The figure shows three views and two pictorial views of one solid part (mm, origin at its lowest corner). Answer the questions. A direction names the side the tool comes from. Round coordinates to 2 decimals unless told otherwise and drop trailing zeros. Loops run counter-clockwise (first coordinate to the right, second up) from the corner with the lowest first, then second, coordinate; pieces in that order, holes last. Notation, with made-up numbers: (-27.5, 84.5) -> (11.5, 84.5) arc R26 cw to (11.5, 110.5) -> close; hole circle Ø1 at (29.25, -18). An arc over 180 degrees is marked (long way). Use a Markdown table: item, result. Add a question column.
Q1. For a pull along Y with two mould halves and no side action, classify the marked faces 1, 2 and 3 as released by +Y, released by -Y, zero draft, split by the parting line, or undercut.
Q2. Given pin 1 Ø1.5 at (x, z) = (2.5, 4) entering from -Y, flat-ended and moving along its own axis, determine where the tip first touches the part or whether it passes through.
Q3. Section A-A on y = 2.4 is taken. Give the vertices of the cut face in (x, z).
Q4. Which of the six approach directions +Z, -Z, +X, -X, +Y, -Y give full straight-line access (tool end or side, diameter ignored) to the marked faces 4 and 5?
Q5. Section C-C on z = 8.75 is taken. Give the vertices of the cut face in (x, y).
Q6. Section B-B on x = 3.15 is taken. Give the vertices of the cut face in (y, z).
Q7. Section D-D on x = 4.05 is taken. Give the vertices of the cut face in (y, z).
Q8. Consider line 1 (Z direction, x = 1.1, y = 4.2); line 2 (X direction, y = 1.8, z = 10.75); line 3 (Z direction, x = 2.2, y = 2.6). Determine where each line is inside the solid, lowest interval first.
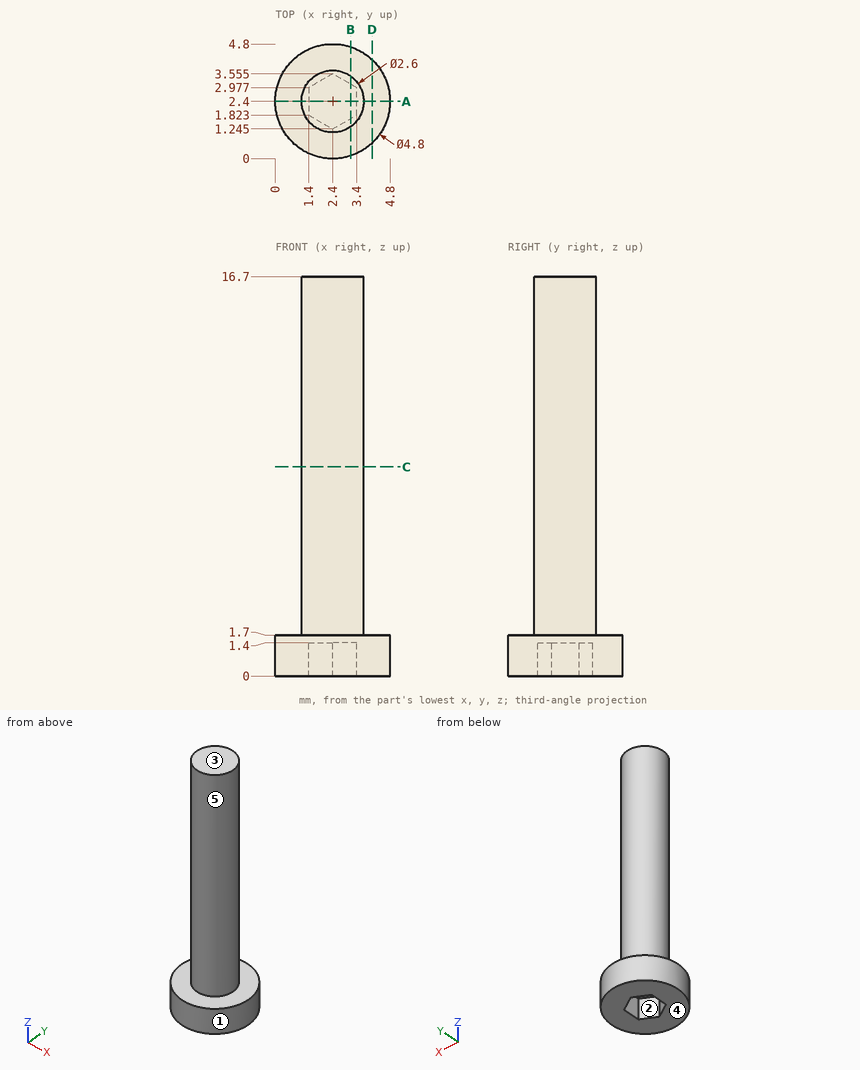
Checked values:
| question | item | result |
|---|---|---|
| 1 | face 1 | split by the parting line |
| 1 | face 2 | undercut |
| 1 | face 3 | zero draft |
| 2 | pin 1 | stops at y = 1.1 |
| 3 | outline | (0, 0) -> (1.4, 0) -> (1.4, 1.4) -> (3.4, 1.4) -> (3.4, 0) -> (4.8, 0) -> (4.8, 1.7) -> (3.7, 1.7) -> (3.7, 16.7) -> (1.1, 16.7) -> (1.1, 1.7) -> (0, 1.7) -> close |
| 4 | face 4 | -Z, +X, -X, +Y, -Y |
| 4 | face 5 | +Z |
| 5 | outline | circle Ø2.6 at (2.4, 2.4) |
| 6 | outline | (0.12, 0) -> (1.68, 0) -> (1.68, 1.4) -> (3.12, 1.4) -> (3.12, 0) -> (4.68, 0) -> (4.68, 1.7) -> (3.46, 1.7) -> (3.46, 16.7) -> (1.34, 16.7) -> (1.34, 1.7) -> (0.12, 1.7) -> close |
| 7 | outline | (0.66, 0) -> (4.14, 0) -> (4.14, 1.7) -> (0.66, 1.7) -> close |
| 8 | line 1 | z = 0 to 1.7 |
| 8 | line 2 | x = 1.25 to 3.55 |
| 8 | line 3 | z = 1.4 to 16.7 |
